CAD build for the part. Positions are in the model's coordinates, mm. A direction names the side the tool comes from. Coordinates: 2 decimals unless noted, no trailing zeros. Loops run counter-clockwise (first coordinate to the right, second up) from the corner with the lowest first, then second, coordinate; pieces in that order, holes last. Notation, with made-up numbers: (83, 56) -> (131, 56) arc R20 cw to (131, 68) -> close; hole circle Ø2 at (54, 23). An arc over 180 degrees is marked (long way). Write each question's results on one line, items separated by ' | '.
```python
from build123d import *

# Parameters (mm, degrees)
F3_D = 19
F5_D = 5.5


with BuildPart() as f1:
    # F0 (on Right) → F1 (revolve)
    with BuildSketch(Plane.YZ):
        Polygon((-6, -18), (-6, 0), (-50, 0), (-50, -9), (-12, -9), (-12, -18), align=None)
    revolve(axis=Axis((0, 0, -9.1057028621), (0, 0, -1)))

    # F3 (through all)
    with Locations(Plane.XY):
        with Locations((0, 0)):
            Hole(F3_D / 2)

    # F5 (through all)
    with Locations(Plane.XY):
        with Locations((-15.112143296, -8.725), (0, 17.45), (15.112143296, -8.725)):
            Hole(F5_D / 2)


solid = f1.part
```
Q1. Cut at C-C on z = -7.5. Write the cut outline in (x, y) (3 decimals).
Results are:
outline: circle Ø100 at (0, 0); hole circle Ø5.5 at (-15.112, -8.725); hole circle Ø19 at (0, 0); hole circle Ø5.5 at (0, 17.45); hole circle Ø5.5 at (15.112, -8.725)
Q2. Cut at B-B on y = 0. Write the cut outline in (x, z), and give its area (3 significant figures).
Results are:
outline: (-50, -9) -> (-12, -9) -> (-12, -18) -> (-9.5, -18) -> (-9.5, 0) -> (-50, 0) -> close; (9.5, -18) -> (12, -18) -> (12, -9) -> (50, -9) -> (50, 0) -> (9.5, 0) -> close | area: 774 mm^2
Q3. Cut at D-D on y = 17.45. Write the cut outline in (x, z), and give its area (3 significant figures).
Results are:
outline: (-46.86, -9) -> (-2.75, -9) -> (-2.75, 0) -> (-46.86, 0) -> close; (2.75, -9) -> (46.86, -9) -> (46.86, 0) -> (2.75, 0) -> close | area: 794 mm^2
Q4. Cut at A-A on x = 0. Write the cut outline in (y, z).
Results are:
outline: (-50, -9) -> (-12, -9) -> (-12, -18) -> (-9.5, -18) -> (-9.5, 0) -> (-50, 0) -> close; (9.5, -18) -> (12, -18) -> (12, -9) -> (14.7, -9) -> (14.7, 0) -> (9.5, 0) -> close; (20.2, -9) -> (50, -9) -> (50, 0) -> (20.2, 0) -> close
Q5. Which spindle directions (+Z, -Z, +X, -X, +Y, -Y) get a long thin tool onto all of the face, cutting with end or side? Do faces 4 (the flat face through (10, -10, -9)), 5 (the flat face through (-4, -9, -18)). Say none if no direction does.
Results are:
face 4: -Z | face 5: -Z, +X, -X, +Y, -Y
Q6. Drop flat-ended pins along their axis: pin 1 (5 mm diameter, centred on y = 12, z = -5, fed in from -X); pin 2 (7 mm diameter, centred on x = -15.11, y = -8.72, fed in from -Z); pin 3 (17 mm diameter, centred on x = 0, y = 0, fed in from +Z); pin 4 (5 mm diameter, centred on x = -37.5, z = -8, fed in from -Y). Give the stop position or say it passes through.
Results are:
pin 1: x = -49.09 | pin 2: z = -9 | pin 3: through | pin 4: y = -35.71
Q7. Wall check: L1, parallel to Y at x = 0, z = -4; L2, parallel to Z at x = 18, y = -18; L3, parallel to Y at x = -6.5, z = -8.5. Give the ranges that are in metal, low to high. Write a range as from..to.
Results are:
L1: -50..-9.5, 9.5..14.7, 20.2..50 | L2: -9..0 | L3: -49.58..-6.93, 6.93..49.58
Q8. Pull direction Y, two halves, no side cores. Call faces 1 (the flat face through (10, -1, 0)), 2 (the cylindrical face through (-0.53, 11.99, -13.56)), 3 (the cylindrical face through (12.572, -9.778, -4.563)): +Y half, -Y half, draft (parallel to the pull), parting line (faces both ways), or undercut.
Results are:
face 1: draft | face 2: parting line | face 3: undercut
